Geometry: final body of the model. Coordinates: model frame, mm. A direction names the side the tool comes from. Round coordinates to 2 decimals unless told otherwise and drop trailing zeros. Loops run counter-clockwise (first coordinate to the right, second up) from the corner with the lowest first, then second, coordinate; pieces in that order, holes last. Notation, with made-up numbers: (-29.5, 16) - (15.5, 16) arc R13 ccw to (15.5, 31) - close; hole circle Ø9 at (0, 46). An arc over 180 degrees is marked (long way). Return JSON: item names as keys, results as strings. Group by question number.
1. Material intervals for probe 1 along Y at (x, z) = (-17, -15) (3 decimals); probe 2 along Z at (x, y) = (-12.5, 32.5); probe 3 along X at (y, z) = (177, -50), sorted ascending.
2. Section A-A on z = 35.5. Return loops of the section in (x, y) (3 decimals), and give its area (3 significant figures).
3. Draft query along Y for faces 3 (the face through (3, -5, -73)), 4 (the face through (-17, 360.865, -18)), 5 (the face through (3, 5, -69.58)). Return one class per face: +Y half, -Y half, draft (parallel to the pull), parting line (faces both ways), or undercut.
4. First-contact query: pin 1 Ø1 at (x, y) = (-18.5, -98) entering from +Z; pin 2 Ø5 at (x, y) = (3.42, 320.865) entering from +Z; pin 3 Ø2 at (x, y) = (-4.5, -213.5) entering from -Z. Flat tips, straight axial feed; report the tip coordinate or a pass-through.
5. Section B-B on y = -199.5. Return loops of the section in (x, z), and give its area (3 significant figures).
6. Section C-C on z = -55. Return loops of the section in (x, y) (3 decimals).
7. Set-up query: faces 1 (the face through (-16.58, 25, -48)), 2 (the face through (-17, -360.865, -18)). Return all of +Z, -Z, +X, -X, +Y, -Y with unobstructed straight access to the full face (end or side cutting, diameter ignored); none if empty.
from build123d import *

# Parameters (mm, degrees)
F1_DEPTH = 360.865
F2_W     = 599.73
F2_H     = 120.6
F3_DEPTH = 40.001
F4_R     = 10
F5_R     = 5
F7_D     = 6.6
F8_R     = 4.5
F9_DEPTH = 5
F10_D    = 4.2
F12_D    = 5.5


with BuildPart() as f1:
    # F0 (on Front) → F1 (new body, symmetric)
    with BuildSketch(Plane.XZ):
        with BuildLine():
            Line((-16.58, 73), (-20, 73))
            Line((-20, 73), (-20, -66.16))
            ThreePointArc((-20, -66.16), (-17.9966103833, -70.9966103833), (-13.16, -73))
            Line((-13.16, -73), (20, -73))
            Line((20, -73), (20, -69.58))
            Line((20, -69.58), (-13.16, -69.58))
            ThreePointArc((-13.16, -69.58), (-15.5783051917, -68.5783051917), (-16.58, -66.16))
            Line((-16.58, -66.16), (-16.58, 73))
        make_face()
    extrude(amount=F1_DEPTH, both=True)

    # F2 (on face) → F3 (cut, through all)
    with BuildSketch(Plane(origin=(-20, 0, 0), x_dir=(0, -1, 0), z_dir=(-1, 0, 0))):
        with Locations((0, 12.7)):
            Rectangle(F2_W, F2_H)
    extrude(amount=-F3_DEPTH, mode=Mode.SUBTRACT)

    # F4
    f4_edges = [f1.edges().sort_by_distance(p)[0] for p in [
        (-18.29, 299.865, -47.6),
        (-18.29, -299.865, -47.6),
    ]]
    fillet(f4_edges, radius=F4_R)

    # F5
    f5_edges = [f1.edges().sort_by_distance(p)[0] for p in [
        (20, -360.865, -71.29),
        (20, 360.865, -71.29),
        (-18.29, -360.865, 73),
        (-18.29, -299.865, 73),
        (-18.29, 299.865, 73),
        (-18.29, 360.865, 73),
    ]]
    fillet(f5_edges, radius=F5_R)

    # F7 (through all)
    with Locations(Plane(origin=(-20, 0, 0), x_dir=(0, -1, 0), z_dir=(-1, 0, 0))):
        with Locations((-313.365, -15.5), (-353.365, -15.5), (-313.365, 49.5), (-353.365, 49.5), (313.365, 49.5), (353.365, 49.5), (353.365, -15.5), (313.365, -15.5)):
            Hole(F7_D / 2)

    # F8 (on face) → F9 (join)
    with BuildSketch(Plane.XY.offset(-69.58)):
        with Locations((3.42, 320.865)):
            Circle(F8_R)
        with Locations((3.42, 19.995)):
            Circle(F8_R)
        with Locations((3.42, -19.995)):
            Circle(F8_R)
        with Locations((3.42, -320.865)):
            Circle(F8_R)
        with Locations((3.42, -280.865)):
            Circle(F8_R)
        with Locations((3.42, 280.865)):
            Circle(F8_R)
    extrude(amount=-F9_DEPTH)

    # F10 (through all)
    with Locations(Plane.XY.offset(-69.58)):
        with Locations((3.42, -320.865), (3.42, -19.995), (3.42, 19.995), (3.42, 320.865), (3.42, 280.865), (3.42, -280.865)):
            Hole(F10_D / 2)

    # F12 (through all)
    with Locations(Plane(origin=(-20, 0, 0), x_dir=(0, -1, 0), z_dir=(-1, 0, 0))):
        with Locations((-321.365, 67), (321.365, 67)):
            Hole(F12_D / 2)


solid = f1.part
Taken from the geometry:
{
 "1": {"probe 1": "-360.865 to -356.627, -350.103 to -316.627, -310.103 to -299.865, 299.865 to 310.103, 316.627 to 350.103, 356.627 to 360.865", "probe 2": "-73 to -69.58", "probe 3": "-20 to -16.58"},
 "2": {"outline": "(-20, -360.865) - (-16.58, -360.865) - (-16.58, -299.865) - (-20, -299.865) - close; (-20, 299.865) - (-16.58, 299.865) - (-16.58, 360.865) - (-20, 360.865) - close", "area": "417 mm2"},
 "3": {"face 3": "undercut", "face 4": "+Y half", "face 5": "draft"},
 "4": {"pin 1": "z = -47.6", "pin 2": "z = -69.58", "pin 3": "z = -73"},
 "5": {"outline": "(-20, -66.16) arc R6.84 ccw to (-13.16, -73) - (20, -73) - (20, -69.58) - (-13.16, -69.58) arc R3.42 cw to (-16.58, -66.16) - (-16.58, -47.6) - (-20, -47.6) - close", "area": "204 mm2"},
 "6": {"outline": "(-20, -360.865) - (-16.58, -360.865) - (-16.58, 360.865) - (-20, 360.865) - close"},
 "7": {"face 1": "+Z, +X, +Y, -Y", "face 2": "+Z, -Z, +X, -X, -Y"}
}
